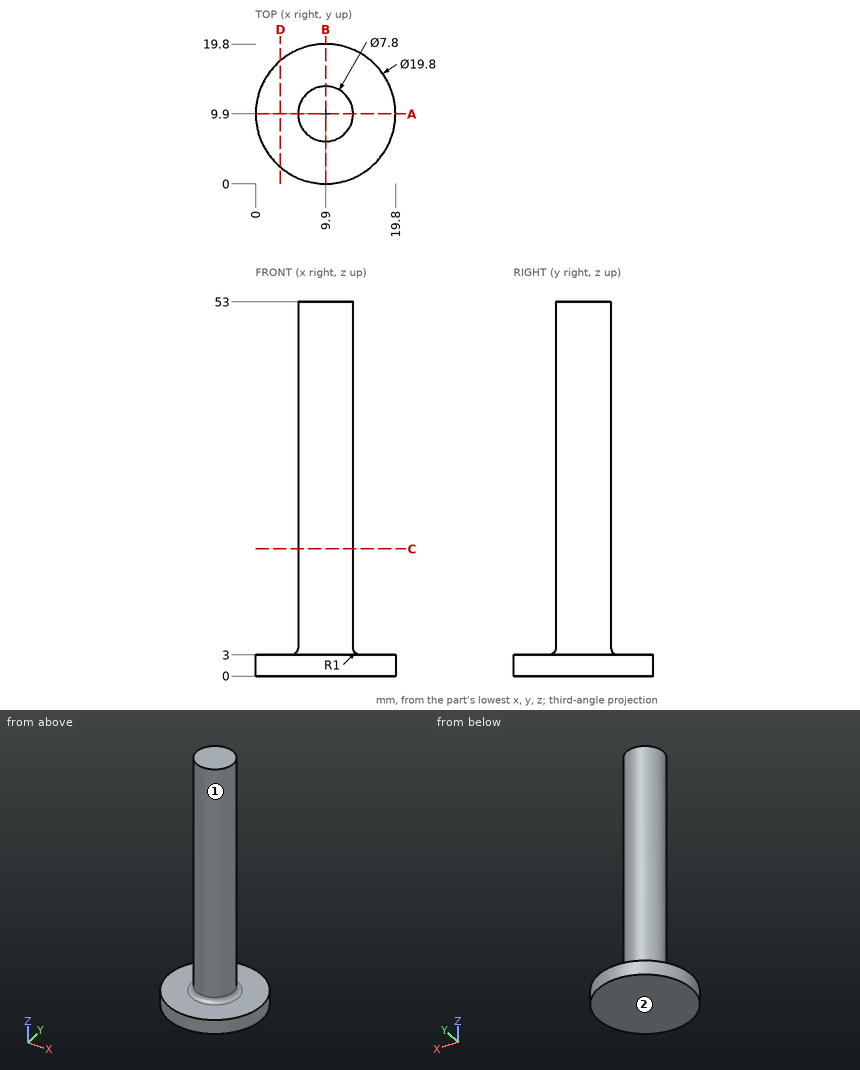
Drawing for the job (mm, zero at the part's lowest x, y, z). A direction names the side the tool comes from. Round coordinates to 2 decimals unless told otherwise and drop trailing zeros. Loops run counter-clockwise (first coordinate to the right, second up) from the corner with the lowest first, then second, coordinate; pieces in that order, holes last. Notation, with made-up numbers: (-18, -3.5) - (-7, -3.5) arc R24 ccw to (-7, 9.5) - close; hole circle Ø9 at (-32.5, 36.5). An arc over 180 degrees is marked (long way). Return JSON: item names as keys, results as strings. Group by question number.
Q1. Band-saw the part on C-C on z = 18. Give the cut face in (x, y), plus the area to 3 significant figures.
Q2. Band-saw the part on A-A on y = 9.9. Give the cut face in (x, z), plus the area to 3 significant figures.
Q3. Tool access for the marked faces 1 and 2: list every direction of +Z, -Z, +X, -X, +Y, -Y with a clear straight run to the whole face (end or side of a thin tool).
Q4. Flat gauge pins, fed straight in: pin 1 Ø1 at (x, y) = (8, 16.5) entering from +Z; pin 2 Ø2 at (y, z) = (12, 12.5) entering from -X; pin 3 Ø8 at (x, z) = (3.5, 19) entering from -Y. Where does each tip first touch, or does it go through?
Q5. Band-saw the part on D-D on x = 3.5. Give the cut face in (y, z).
Q6. Drill centre lines: line 1 along Z through (x, y) = (4.5, 2.75); line 2 along Y through (x, z) = (10, 23); line 3 along X through (y, z) = (7.5, 47.5). Where is each one in solid material? Low to high. Write a range as [from, to].
Solutions:
{
 "1": {"outline": "circle Ø7.8 at (9.9, 9.9)", "area": "47.8 mm^2"},
 "2": {"outline": "(0, 0) - (19.8, 0) - (19.8, 3) - (14.8, 3) arc R1 cw to (13.8, 4) - (13.8, 53) - (6, 53) - (6, 4) arc R1 cw to (5, 3) - (0, 3) - close", "area": "450 mm^2"},
 "3": {"face 1": "+Z", "face 2": "-Z, +X, -X, +Y, -Y"},
 "4": {"pin 1": "stops at z = 3", "pin 2": "stops at x = 6.16", "pin 3": "stops at y = 6.83"},
 "5": {"outline": "(2.35, 0) - (17.45, 0) - (17.45, 3) - (2.35, 3) - close"},
 "6": {"line 1": "z = [0, 3]", "line 2": "y = [6, 13.8]", "line 3": "x = [6.83, 12.97]"}
}
